Can you work these out from the drawing? Everything is in mm from the part's minimum corner. Coordinates: 2 decimals unless noted, no trailing zeros. Write each loop counter-clockwise with the first axis right and the second up, starting at its lowest first coordinate (ties: lowest second). Pieces come first, ordered by that corner, then holes. Notation, with made-up numbers: M 58.25,78 L 76.25,78 A8 ccw 76.25,92 Z; hole C 19,33 d7. An arc over 180 degrees is marked long. Answer as a JSON object with one key per item and string values. Group by question number.
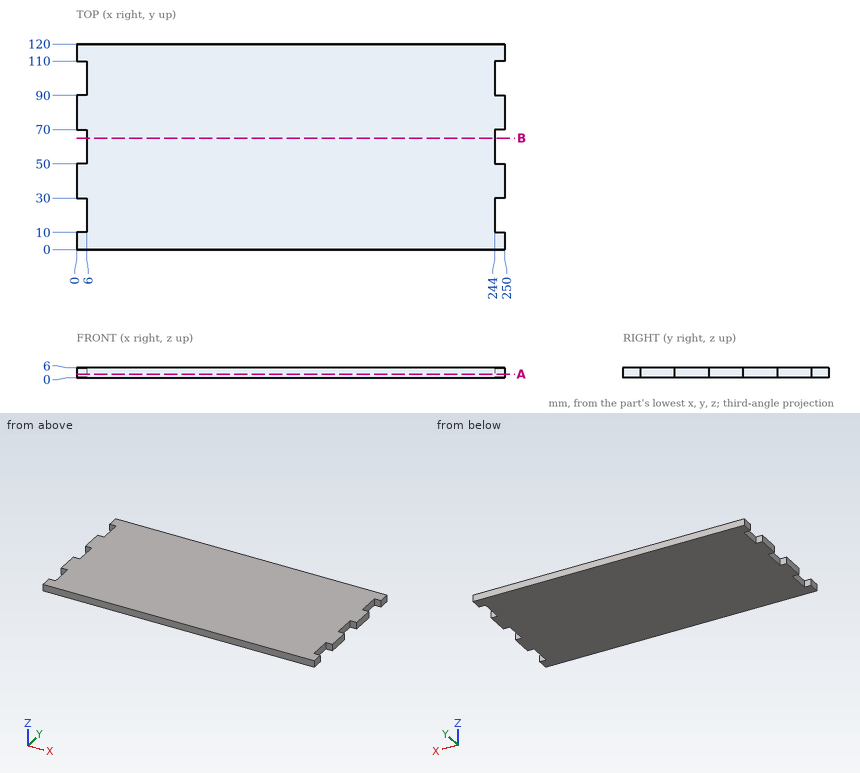
Q1. Will these pins go through, and if not, where does the flat tip stop? pin 1 (3 mm diameter, centred on y = 59, z = 3.5, fed in from +X); pin 2 (1.8 mm diameter, centred on y = 20.5, z = 4, fed in from -X).
Q2. Please list where this line runs through material, in increasing order: L1, parallel to X at y = 50.5, z = 2.3.
Q3. If we section it at B-B on y = 65: List the corners of the cut face in (x, z) for me.
Q4. If we section it at A-A on z = 2.25: List the corners of the cut face in (x, y) for me, and give its area (3 significant figures).
Reply:
{
 "1": {"pin 1": "x = 244", "pin 2": "x = 6"},
 "2": {"L1": "6 to 244"},
 "3": {"outline": "M 6,0 L 244,0 L 244,6 L 6,6 Z"},
 "4": {"outline": "M 0,0 L 250,0 L 250,10 L 244,10 L 244,30 L 250,30 L 250,50 L 244,50 L 244,70 L 250,70 L 250,90 L 244,90 L 244,110 L 250,110 L 250,120 L 0,120 L 0,110 L 6,110 L 6,90 L 0,90 L 0,70 L 6,70 L 6,50 L 0,50 L 0,30 L 6,30 L 6,10 L 0,10 Z", "area": "29,300 mm^2"}
}
